Could you check a few things on this model? Use its own coordinates, in mm. A direction names the side the tool comes from. Give positions to 0.01 mm unless a question says otherwise; leave off trailing zeros. Order: outer loops, then holes, each group sorted by start corner. A loop starts at its lowest first (then second) coordinate and runs counter-clockwise, first axis right, second up.
(1) Imagine slicing it at A-A, the plane y = -0.5. Write out the boundary of the cut face in (x, z), then the cut area to 3 significant figures.
(2) If I drill on probe 1 along Y at (x, z) = (14.5, 0.45); probe 2 along X at (y, z) = (-2.25, 1.5); probe 3 along Y at (x, z) = (-14, 2.5), over which ranges is the centre line in solid material (lowest first)?
(3) Imagine slicing it at B-B, the plane x = 1. Write out the boundary of the cut face in (y, z), then the cut area to 3 significant figures.
(4) Imagine slicing it at D-D, the plane y = 1.5. Write out the boundary of the cut face in (x, z), then the cut area to 3 significant figures.
(5) Imagine slicing it at C-C, the plane z = 2.75. State how many separate pieces and enclosed holes the cut face has, then the cut area to 3 significant figures.
(6) If we mould it in two halves opening along Y, with no side actions, what happens to faces 3 (the cylindrical face through (-11.813, 0.015, 1.726)), 4 (the flat face through (0, 3, 3.5)), 5 (the flat face through (0, -5, 2))? For each: released by +Y, released by -Y, zero draft, split by the parting line, or undercut.
(7) On a 3-axis mill with a long thin cutter (end or side, diameter ignored), from which of +Z, -Z, +X, -X, +Y, -Y can I reach the whole of each face in a straight line? I mean faces 1 (the flat face through (2.386, 1.387, 1.726)), 2 (the flat face through (20, 0, 2)). Say none if no direction works.
Autodesk Inventor part; units mm, degrees
ref_plane "YZ Plane" through (0, 0, 0) normal (1, 0, 0) x (0, 1, 0)
ref_plane "XZ Plane" through (0, 0, 0) normal (0, 1, 0) x (-1, 0, 0)
ref_plane "XY Plane" through (0, 0, 0) normal (0, 0, 1) x (1, 0, 0)
sketch "スケッチ1" plane through (0, 0, 0) normal (0, 0, 1) x (1, 0, 0)
  line L0 (-20, -5) -> (20, -5)
  line L1 (20, -5) -> (20, 5)
  line L2 (20, 5) -> (-20, 5)
  line L3 (-20, 5) -> (-20, -5)
  line L4 (-20, -5) -> (20, 5) construction
  line L5 (20, -5) -> (-20, 5) construction
  circle A0 centre (-15, 0) radius 1.55
  circle A1 centre (0, 0) radius 1.55
  line L6 (0, 0) -> (0, 5) construction
  line L7 (-12.5995, 5) -> (4.4005, 5) construction
  line L8 (-8.5, -4) -> (8.5, -4) construction
  line L9 (-13.4065, -2.76) -> (-16.5935, -2.76)
  line L10 (-16.5935, -2.76) -> (-18.187, 0)
  line L11 (-18.187, 0) -> (-16.5935, 2.76)
  line L12 (-16.5935, 2.76) -> (-13.4065, 2.76)
  line L13 (-13.4065, 2.76) -> (-11.813, 0)
  line L14 (-11.813, 0) -> (-13.4065, -2.76)
  circle A2 centre (-17.137, 0) radius 1.05
  circle A3 centre (-16.0685, -1.8507) radius 1.05
  circle A4 centre (-13.9315, -1.8507) radius 1.05
  circle A5 centre (-12.863, 0) radius 1.05
  circle A6 centre (-13.9315, 1.8507) radius 1.05
  circle A7 centre (-16.0685, 1.8507) radius 1.05
  circle A8 centre (15, 0) radius 1.55
  line L15 (13.4065, -2.76) -> (16.5935, -2.76)
  line L16 (16.5935, -2.76) -> (18.187, 0)
  line L17 (18.187, 0) -> (16.5935, 2.76)
  line L18 (16.5935, 2.76) -> (13.4065, 2.76)
  line L19 (13.4065, 2.76) -> (11.813, 0)
  line L20 (11.813, 0) -> (13.4065, -2.76)
  circle A9 centre (17.137, 0) radius 1.05
  circle A10 centre (16.0685, -1.8507) radius 1.05
  circle A11 centre (13.9315, -1.8507) radius 1.05
  circle A12 centre (12.863, 0) radius 1.05
  circle A13 centre (13.9315, 1.8507) radius 1.05
  circle A14 centre (16.0685, 1.8507) radius 1.05
  circle A15 centre (-15, 0) radius 5 construction
  line L21 (1.5935, -2.76) -> (-1.5935, -2.76)
  line L22 (-1.5935, -2.76) -> (-3.187, 0)
  line L23 (-3.187, 0) -> (-1.5935, 2.76)
  line L24 (-1.5935, 2.76) -> (1.5935, 2.76)
  line L25 (1.5935, 2.76) -> (3.187, 0)
  line L26 (3.187, 0) -> (1.5935, -2.76)
  circle A16 centre (-2.137, 0) radius 1.05
  circle A17 centre (-1.0685, -1.8507) radius 1.05
  circle A18 centre (1.0685, -1.8507) radius 1.05
  circle A19 centre (2.137, 0) radius 1.05
  circle A20 centre (1.0685, 1.8507) radius 1.05
  circle A21 centre (-1.0685, 1.8507) radius 1.05
  point P0 (-16.5935, -2.76)
  point P1 (-13.4065, -2.76)
  point P2 (-11.813, 0)
  point P3 (-13.4065, 2.76)
  point P4 (-16.5935, 2.76)
  point P5 (16.5935, -2.76)
  point P6 (13.4065, -2.76)
  point P7 (11.813, 0)
  point P8 (13.4065, 2.76)
  point P9 (16.5935, 2.76)
  point P10 (-1.5935, -2.76)
  point P11 (1.5935, -2.76)
  point P12 (3.187, 0)
  point P13 (1.5935, 2.76)
  dimension "d19" = 2.1
  dimension "d1" = 3.1
  dimension "d4" = 15
  dimension "d5" = 10
  dimension "d20" = 5.52
  dimension "d23" = 360
  dimension "d33" = 360
extrude "押し出し1" add sketch "スケッチ1" along normal blind 3.5
properties part number "胴体_サブフレーム_1_2" material "アセタール樹脂、黒"
Answer block:
1. outline: (-20, 0) - (-18.06, 0) - (-18.06, 3.5) - (-20, 3.5) - close; (-11.94, 0) - (-3.06, 0) - (-3.06, 3.5) - (-11.94, 3.5) - close; (3.06, 0) - (11.94, 0) - (11.94, 3.5) - (3.06, 3.5) - close; (18.06, 0) - (20, 0) - (20, 3.5) - (18.06, 3.5) - close
1. area: 75.7 mm2
2. probe 1: y = -5 to -2.76, 2.76 to 5
2. probe 2: x = -20 to -17.04, -12.96 to -2.04, 2.04 to 12.96, 17.04 to 20
2. probe 3: y = -5 to -2.9, 2.9 to 5
3. outline: (-5, 0) - (-2.9, 0) - (-2.9, 3.5) - (-5, 3.5) - close; (2.9, 0) - (5, 0) - (5, 3.5) - (2.9, 3.5) - close
3. area: 14.7 mm2
4. outline: (-20, 0) - (-17.32, 0) - (-17.32, 3.5) - (-20, 3.5) - close; (-12.68, 0) - (-2.32, 0) - (-2.32, 3.5) - (-12.68, 3.5) - close; (2.32, 0) - (12.68, 0) - (12.68, 3.5) - (2.32, 3.5) - close; (17.32, 0) - (20, 0) - (20, 3.5) - (17.32, 3.5) - close
4. area: 91.3 mm2
5. separate pieces: 1
5. enclosed holes: 3
5. area: 317 mm2
6. face 3: undercut
6. face 4: zero draft
6. face 5: released by -Y
7. face 1: +Z, -Z
7. face 2: +Z, -Z, +X, +Y, -Y
